from build123d import *

# Parameters (mm, degrees)
BASE_DEPTH                 = 4
SKETCH2_W                  = 45
SKETCH2_H                  = 40
TPS_STANDOFF_DEPTH         = 4
SKETCH4_R                  = 1.925
TPS_SCREW_HOLES_DEPTH      = 8
MOUNTING_SCREW_HOLES_DEPTH = 4
SKETCH7_R                  = 10
SKETCH7_R_2                = 7.5
O_RING_CUT_DEPTH           = 2.5
CHAMFER1_SIZE              = 4
CHAMFER3_SIZE              = 0.25
CUT_EXTRUDE3_DEPTH         = 90.532117142
CUT_EXTRUDE3_DEPTH_BACK    = 90.532117142
FILLET4_R                  = 11


with BuildPart() as part:
    # Sketch1 → Base (new body)
    with BuildSketch(Plane(origin=(0, 0, 0), x_dir=(1, 0, 0), z_dir=(0, 1, 0))):
        Polygon((-5, 40), (65, 40), (80, 0), (60, 0), (0, 0), (-15, 40), align=None)
    extrude(amount=BASE_DEPTH)

    # Sketch2 → TPS Standoff (add)
    with BuildSketch(Plane(origin=(0, 4, 0), x_dir=(1, 0, 0), z_dir=(0, 1, 0))):
        with Locations((32.5, 20)):
            Rectangle(SKETCH2_W, SKETCH2_H)
    extrude(amount=TPS_STANDOFF_DEPTH)

    # Sketch4 → TPS Screw Holes (cut)
    with BuildSketch(Plane(origin=(0, 8, 0), x_dir=(1, 0, 0), z_dir=(0, 1, 0))):
        with Locations(Location((48.5, 20, 0), (0, 0, 270))):
            Circle(SKETCH4_R)
        with Locations(Location((16.5, 20, 0), (0, 0, 270))):
            Circle(SKETCH4_R)
    extrude(amount=-TPS_SCREW_HOLES_DEPTH, mode=Mode.SUBTRACT)

    # Sketch5 → Mounting Screw Holes (cut)
    with BuildSketch(Plane(origin=(0, 4, 0), x_dir=(1, 0, 0), z_dir=(0, 1, 0))):
        with BuildLine():
            ThreePointArc((-1.640188927, 34.9), (-3.174301135, 30.719456076), (-4.19857154, 26.385714286))
            ThreePointArc((-4.19857154, 26.385714286), (-2.367593585, 23.783307759), (0.234812942, 25.614285714))
            ThreePointArc((0.234812942, 25.614285714), (1.135345982, 29.424488228), (2.484129198, 33.1))
            ThreePointArc((2.484129198, 33.1), (1.321970135, 36.062159063), (-1.640188927, 34.9))
        make_face()
        with BuildLine():
            ThreePointArc((66.640188927, 5.1), (68.174301135, 9.280543924), (69.19857154, 13.614285714))
            ThreePointArc((69.19857154, 13.614285714), (67.367593585, 16.216692241), (64.765187058, 14.385714286))
            ThreePointArc((64.765187058, 14.385714286), (63.864654018, 10.575511772), (62.515870802, 6.9))
            ThreePointArc((62.515870802, 6.9), (63.678029865, 3.937840937), (66.640188927, 5.1))
        make_face()
    extrude(amount=-MOUNTING_SCREW_HOLES_DEPTH, mode=Mode.SUBTRACT)

    # Sketch6 → TPS Shaft Bore Cut (revolve, cut)
    with BuildSketch(Plane.YZ.offset(32.5)):
        Polygon((8, -20), (0, -20), (0, -24.15), (5.5, -24.15), (5.5, -27.55), (8, -27.55), align=None)
    revolve(axis=Axis((32.5, 8, -20), (0, 1, 0)), mode=Mode.SUBTRACT)

    # Sketch7 → O-Ring Cut (cut)
    with BuildSketch(Plane.XZ):
        with Locations(Location((32.5, -20, 0), (0, 0, 270))):
            Circle(SKETCH7_R)
        with Locations(Location((32.5, -20, 0), (0, 0, 270))):
            Circle(SKETCH7_R_2, mode=Mode.SUBTRACT)
    extrude(amount=-O_RING_CUT_DEPTH, mode=Mode.SUBTRACT)

    # Chamfer1
    chamfer1_edges = [part.edges().sort_by_distance(p)[0] for p in [
        (55, 4, -20),
        (10, 4, -20),
    ]]
    chamfer(chamfer1_edges, length=CHAMFER1_SIZE - 0.0001)  # a hair under: the kernel refuses the full size

    # Chamfer3
    chamfer3_edges = [part.edges().sort_by_distance(p)[0] for p in [
        (32.5, 8, 0),
        (32.5, 8, -40),
        (48.5, 8, -21.925),
        (16.5, 8, -21.925),
        (32.5, 8, -12.45),
        (32.5, 5.5, -15.85),
    ]]
    chamfer(chamfer3_edges, length=CHAMFER3_SIZE)

    # Sketch9 → Cut-Extrude3 (cut, two sides: drawn at the far end of the back side and taken through both)
    with BuildSketch(Plane(origin=(0, 4, 0), x_dir=(1, 0, 0), z_dir=(0, 1, 0)).offset(-CUT_EXTRUDE3_DEPTH_BACK)):
        Polygon((6, 0), (-9, 24), (0, 0), align=None)
        Polygon((59, 40), (65, 40), (74, 16), align=None)
    extrude(amount=CUT_EXTRUDE3_DEPTH + CUT_EXTRUDE3_DEPTH_BACK, mode=Mode.SUBTRACT)

    # Fillet4
    fillet4_edges = [part.edges().sort_by_distance(p)[0] for p in [
        (-15, 2, -40),
        (80, 2, 0),
        (-9, 2, -24),
        (74, 2, -16),
    ]]
    fillet(fillet4_edges, radius=FILLET4_R)


solid = part.part
Input: part model. Units: mm. Frame: model coordinates. A direction names the side the tool comes from. Coordinates: 2 decimals unless noted, no trailing zeros. Order: outer loops, then holes, each group sorted by start corner. A loop starts at its lowest first (then second) coordinate and runs counter-clockwise, first axis right, second up. Notation, with made-up numbers: M -6.75,72.25 L 38.25,72.25 A27 cw 38.25,101.25 Z; hole C -11.5,79.25 d6. An arc over 180 degrees is marked long. Answer as CSV lines item,"result".
1. Section A-A (y = 1). Return the cut outline in (x, z) (3 decimals), then the cut area to 3 significant figures.
Reported:
outline,"M -9.427,-25.138 A11 ccw 0.873,-40 L 59,-40 L 73.416,-16.935 A11 ccw 74.387,-14.967 L 74.427,-14.862 A11 ccw 64.127,0 L 6,0 L -8.416,-23.065 A11 ccw -9.387,-25.033 Z; C 32.5,-20 d15; hole M -4.199,-26.386 A37.25 ccw -1.64,-34.9 A2.25 ccw 2.484,-33.1 A32.75 cw 0.235,-25.614 A2.25 ccw Z; hole C 16.5,-20 d3.85; hole C 32.5,-20 d20; hole C 32.5,-20 d8.3; hole C 48.5,-20 d3.85; hole M 62.516,-6.9 A32.75 cw 64.765,-14.386 A2.25 ccw 69.199,-13.614 A37.25 ccw 66.64,-5.1 A2.25 ccw Z"
area,"2,620 mm2"
2. Material intervals for line 1 (X direction, y = 3.35, z = -20) (3 decimals); line 2 (Z direction, x = 32.5, y = 6.15); line 3 (X direction, y = 4.25, z = -21.5), sorted ascending. Write a range as from..to.
Reported:
line 1,"-6.5..14.575, 18.425..28.35, 36.65..46.575, 50.425..71.5"
line 2,"-40..-27.55, -12.45..0"
line 3,"6.25..15.29, 17.71..28.63, 36.37..47.29, 49.71..58.75"
3. Pull-direction query (Z, two-part tool) for faces 4 (the flat face through (57, 6, -20)), 5 (the flat face through (-1.107, 1.972, -11.371)), 6 (the cylindrical face through (63.63, 2.03, -3.96)), 7 (the cylindrical face through (63.88, 2.03, -10.63)); classes: released by +Z, released by -Z, zero draft, split by the parting line, or undercut.
Reported:
face 4,"zero draft"
face 5,"released by +Z"
face 6,"undercut"
face 7,"undercut"
4. First-contact query: P1, Ø16, axis at x = 30, z = -23, coming from the -Y side; P2, Ø3.5, axis at x = 16.5, z = -20, coming from the +Y side; P3, Ø4, axis at x = -1, z = -9, coming from the +Y side; P4, Ø7.5, axis at x = 29.5, z = -22.5, coming from the +Y side. Flat tips, straight axial feed; report the tip coordinate or a pass-through.
Reported:
P1,"y = 0"
P2,"through"
P3,"y = 4"
P4,"y = 7.86"
5. Section B-B (x = 32.5). Return the cut outline in (y, z).
Reported:
outline,"M 0,-40 L 7.75,-40 L 8,-39.75 L 8,-27.8 L 7.75,-27.55 L 5.5,-27.55 L 5.5,-24.4 L 5.25,-24.15 L 0,-24.15 L 0,-27.5 L 2.5,-27.5 L 2.5,-30 L 0,-30 Z; M 0,-15.85 L 5.25,-15.85 L 5.5,-15.6 L 5.5,-12.45 L 7.75,-12.45 L 8,-12.2 L 8,-0.25 L 7.75,0 L 0,0 L 0,-10 L 2.5,-10 L 2.5,-12.5 L 0,-12.5 Z"
6. Access query for faces 1 (the cylindrical face through (25.18, 1.23, -18.37)), 2 (the cylindrical face through (68.156, 2.028, -9.221)), 3 (the flat face through (2, 4, -25)). Directions: +Z, -Z, +X, -X, +Y, -Y. A direction counts if a zero-diameter tool reaches every point of the face in a straight line with its end or side. Return the directions, or none.
Reported:
face 1,"-Y"
face 2,"+Y, -Y"
face 3,"+Z, -Z, -X, +Y"
7. Section D-D (y = 6.75). Return the cut outline in (x, z) (3 decimals).
Reported:
outline,"M 8.75,-40 L 56.25,-40 L 56.25,0 L 8.75,0 Z; hole C 16.5,-20 d3.85; hole C 32.5,-20 d15.1; hole C 48.5,-20 d3.85"
